Autodesk Fusion 360 part; units mm, degrees
sketch "Sketch1" plane through (0, 0, 0) normal (0, 0, 1) x (1, 0, 0)
  line L0 (0, 0) -> (20, 0)
  line L1 (20, 0) -> (20, 20)
  line L2 (20, 20) -> (0, 20)
  line L3 (0, 20) -> (0, 0)
  dimension "d1" = 20
  dimension "d2" = 20
extrude "Extrude1" add sketch "Sketch1" along normal blind 4
sketch "Sketch2" plane through (0, 0, 4) normal (0, 0, 1) x (-1, 0, 0)
  line L0 (0, -20) -> (0, 0)
  line L1 (0, 0) -> (-20, 0)
  line L2 (-20, 0) -> (-20, -20)
  line L3 (-20, -20) -> (0, -20)
  line L4 (-3, -20) -> (-3, 0)
  circle A0 centre (-11.5, -10) radius 2.75
  circle A1 centre (-11.5, -10) radius 5.5
  line L5 (0, -10) -> (-20, -10) construction
  dimension "d5" = 5.5
  dimension "d6" = 11
  dimension "d7" = 3
  dimension "d8" = 3
  dimension "d9" = 3
extrude "Extrude2" cut sketch "Sketch2" against normal up to surface (4 mm away) contours A0
extrude "Extrude3" cut sketch "Sketch2" against normal blind 2 contours A1
extrude "Extrude4" add sketch "Sketch2" along normal blind 18 contours L0 L1 L3 L4
sketch "Sketch3" plane through (3, 0, 0) normal (1, 0, 0) x (0, 1, 0)
  line L0 (0, 4) -> (20, 4)
  line L1 (20, 4) -> (20, 22)
  line L2 (20, 22) -> (0, 22)
  line L3 (0, 22) -> (0, 4)
  line L4 (0, 13) -> (20, 13) construction
  line L5 (10, 22) -> (10, 4) construction
  circle A0 centre (10, 13) radius 6.5
  dimension "d16" = 13
extrude "Extrude5" cut sketch "Sketch3" against normal up to surface (3 mm away) contours A0
sketch "Sketch4" plane through (0, 0, 0) normal (0, 0, -1) x (1, 0, 0)
  circle A0 centre (11.5, -10) radius 2.75
  line L0 (0, 0) -> (0, -20)
  line L1 (0, -20) -> (20, -20)
  line L2 (20, -20) -> (20, 0)
  line L3 (20, 0) -> (0, 0)
  line L4 (0, -10) -> (20, -10) construction
  line L5 (20, -12.5) -> (18.5, -12.5)
  line L6 (18.5, -12.5) -> (18.5, -7.5)
  line L7 (18.5, -7.5) -> (20, -7.5)
  line L8 (10, -20) -> (10, 0) construction
  line L9 (0, -12.5) -> (1.5, -12.5)
  line L10 (1.5, -12.5) -> (1.5, -7.5)
  line L11 (1.5, -7.5) -> (0, -7.5)
  dimension "d19" = 5
  dimension "d20" = 1.5
  dimension "d21" = 7.5
extrude "Extrude6" add sketch "Sketch4" along normal blind 1.5 contours L0 L9 L10 L11 | L2 L5 L6 L7
The listing builds one solid part. Answer for the finished solid, in the listing's coordinates (mm). A direction names the side the tool comes from. Coordinates: 2 decimals unless noted, no trailing zeros. Loops run counter-clockwise (first coordinate to the right, second up) from the corner with the lowest first, then second, coordinate; pieces in that order, holes last. Notation, with made-up numbers: (20.25, -9.75) -> (68.25, -9.75) arc R9 ccw to (68.25, 5.25) -> close; hole circle Ø8 at (50.25, 67). An arc over 180 degrees is marked (long way). Return JSON: item names as keys, results as strings. Group by question number.
(1) Determine the mould class of faces 4 (the flat face through (1, 12.5, -1)), 5 (the cylindrical face through (9, 14.9, 3)), 6 (the cylindrical face through (1.521, 13.494, 18.481)), 7 (the flat face through (3, 17, 13)) for opening direction Y: released by +Y, released by -Y, zero draft, split by the parting line, or undercut.
(2) A cutting plane is placed at C-C on y = 10. Write down the section's boundary in (x, z), and give its area (3 significant figures).
(3) A cutting plane is placed at B-B on x = 11.5. Write down the section's boundary in (y, z).
(4) Find the intervals of material crossed by probe 1 along Z at (x, y) = (2.35, 10); probe 2 along Y at (x, z) = (11.5, 2.55); probe 3 along X at (y, z) = (10, 2.8), in increasing order. Write a range as from..to.
(5) Which of the six approach directions +Z, -Z, +X, -X, +Y, -Y give full straight-line access (tool end or side, diameter ignored) to faces 1 (the flat face through (10, 7, 2)), 2 (the flat face through (19, 7.5, -1)), 3 (the flat face through (18.5, 10, -1))?
(6) A cutting plane is placed at D-D on z = 9. Write down the section's boundary in (x, y), and give its area (3 significant figures).
(7) A cutting plane is placed at A-A on y = 16. Write down the section's boundary in (x, z).
(8) Given pin 1 Ø4 at (y, z) = (17, 11) entering from -X; pin 2 Ø6.5 at (x, y) = (11.5, 10) entering from -Z; pin 3 Ø4 at (y, z) = (5, 14) entering from +X; pin 4 Ø8 at (x, y) = (8, 10.5) entering from +Z, each flat-ended and moving along its own axis, determine where each tip first touches the part or whether it passes through.
The answers:
{
 "1": {"face 4": "released by +Y", "face 5": "undercut", "face 6": "undercut", "face 7": "zero draft"},
 "2": {"outline": "(0, -1.5) -> (1.5, -1.5) -> (1.5, 0) -> (8.75, 0) -> (8.75, 2) -> (6, 2) -> (6, 4) -> (3, 4) -> (3, 6.5) -> (0, 6.5) -> close; (0, 19.5) -> (3, 19.5) -> (3, 22) -> (0, 22) -> close; (14.25, 0) -> (18.5, 0) -> (18.5, -1.5) -> (20, -1.5) -> (20, 4) -> (17, 4) -> (17, 2) -> (14.25, 2) -> close", "area": "66.5 mm^2"},
 "3": {"outline": "(0, 0) -> (7.25, 0) -> (7.25, 2) -> (4.5, 2) -> (4.5, 4) -> (0, 4) -> close; (12.75, 0) -> (20, 0) -> (20, 4) -> (15.5, 4) -> (15.5, 2) -> (12.75, 2) -> close"},
 "4": {"probe 1": "z = 0..6.5, 19.5..22", "probe 2": "y = 0..4.5, 15.5..20", "probe 3": "x = 0..6, 17..20"},
 "5": {"face 1": "+Z", "face 2": "-Z, +X, -X, -Y", "face 3": "-Z, +Y, -Y"},
 "6": {"outline": "(0, 0) -> (3, 0) -> (3, 4.88) -> (0, 4.88) -> close; (0, 15.12) -> (3, 15.12) -> (3, 20) -> (0, 20) -> close", "area": "29.3 mm^2"},
 "7": {"outline": "(0, 0) -> (20, 0) -> (20, 4) -> (3, 4) -> (3, 10.5) -> (0, 10.5) -> close; (0, 15.5) -> (3, 15.5) -> (3, 22) -> (0, 22) -> close"},
 "8": {"pin 1": "stops at x = 0", "pin 2": "stops at z = 0", "pin 3": "stops at x = 3", "pin 4": "stops at z = 4"}
}
